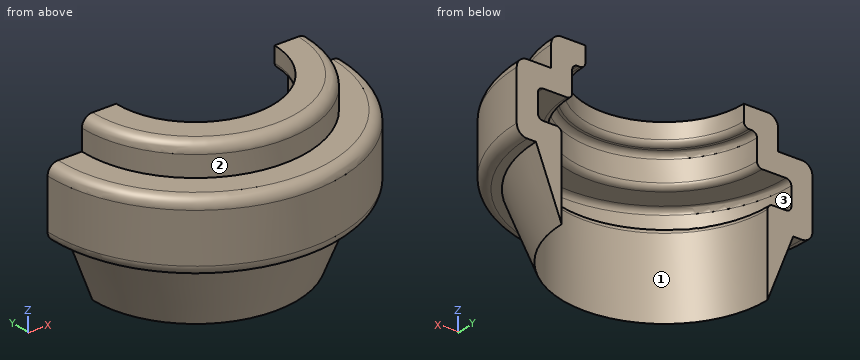
from build123d import *

# Parameters (mm, degrees)
F1_ANGLE = 180
F2_R     = 1
F3_R     = 2


with BuildPart() as f1:
    # F0 (on Front) → F1 (revolve)
    with BuildSketch(Plane.XZ):
        Polygon((21.5, 15.915055), (15, 15.915055), (15, 11.915055), (17.5, 11.915055), (17.5, 5.915055), (24, 5.915055), (24, 0.415055), (19.5, 0.415055), (19.5, -16), (24.362529, -3.584945), (28, -3.584945), (28, 9.915055), (21.5, 9.915055), align=None)
    revolve(axis=Axis((0, 0, -25.149144), (0, 0, -1)), revolution_arc=F1_ANGLE)

    # F2
    f2_edges = [f1.edges().sort_by_distance(p)[0] for p in [
        (0, -17.5, 11.915055),
        (0, -17.5, 5.915055),
        (0, -19.5, 0.415055),
        (0, -24, 5.915055),
        (0, -15, 11.915055),
        (0, -24, 0.415055),
    ]]
    fillet(f2_edges, radius=F2_R)

    # F3
    f3_edges = [f1.edges().sort_by_distance(p)[0] for p in [
        (0, -28, -3.584945),
        (0, -28, 9.915055),
        (0, -21.5, 15.915055),
    ]]
    fillet(f3_edges, radius=F3_R)


solid = f1.part
Verification items for the finished model (mm, model axes). Face numbers are marked on the shaded views. A direction names the side the tool comes from. Give positions to 0.01 mm unless a question says otherwise; leave off trailing zeros. Write each loop counter-clockwise with the first axis right and the second up, starting at its lowest first coordinate (ties: lowest second). Pieces come first, ordered by that corner, then holes. Notation, with made-up numbers: M 62,-11 L 103,-11 A19 cw 103,4 Z; hole C -21,-22.5 d5. An arc over 180 degrees is marked long. Use CSV: the item, a comma, the result in double quotes.
1) Access from +Z, -Z, +X, -X, +Y, -Y to the whole of each face (thin tool, end or side, straight path). Record for the marked faces 1, 2 and 3.
Final values:
face 1,"-Z, +Y"
face 2,"+Z, -Y"
face 3,"+Y"
2) Material ranges on line 1 along X through (y, z) = (-14.5, -5); line 2 along X through (y, z) = (-7.5, 1); line 3 along Z through (x, y) = (2, -16.25), recorded low to high.
Final values:
line 1,"-18.88 to -13.04, 13.04 to 18.88"
line 2,"-26.98 to -22.7, 22.7 to 26.98"
line 3,"11.92 to 15.92"
3) Cross-section at B-B (z = -7.5). Enter the section's corners in (x, y), plus the area to 3 significant figures.
Final values:
outline,"M -22.83,0 A22.83 ccw 22.83,0 L 19.5,0 A19.5 cw -19.5,0 Z"
area,"221 mm²"
4) Cross-section at A-A (x = 0). Enter the section's corners in (y, z), plus the area to 3 significant figures.
Final values:
outline,"M -28,-1.58 A2 ccw -26,-3.58 L -24.36,-3.58 L -19.5,-16 L -19.5,-0.58 A1 ccw -20.5,0.42 L -23,0.42 A1 cw -24,1.42 L -24,4.92 A1 cw -23,5.92 L -18.5,5.92 A1 ccw -17.5,6.92 L -17.5,10.92 A1 cw -16.5,11.92 L -16,11.92 A1 ccw -15,12.92 L -15,15.92 L -19.5,15.92 A2 ccw -21.5,13.92 L -21.5,9.92 L -26,9.92 A2 ccw -28,7.92 Z"
area,"160 mm²"
5) Go/stop test with flat-tipped pins: pin 1 Ø10 at (x, y) = (-21.5, -23.5) entering from -Z; pin 2 Ø5 at (x, z) = (-12.5, -7) entering from -Y; pin 3 Ø4 at (y, z) = (-13.5, 8.5) entering from -X; pin 4 Ø3 at (x, y) = (15.5, -9.5) entering from -Z. Record where each tip stops, or that it passes through.
Final values:
pin 1,"z = -3.39"
pin 2,"y = -21.15"
pin 3,"x = -25.5"
pin 4,"z = -16"
